Part model, mm, in its own coordinate system. Round coordinates to 2 decimals unless told otherwise and drop trailing zeros. Order: outer loops, then holes, each group sorted by start corner. A loop starts at its lowest first (then second) coordinate and runs counter-clockwise, first axis right, second up. Notation, with made-up numbers: (53, -8) -> (63, -8) arc R27 ccw to (63, 18) -> close; hole circle Ø2 at (59, -31.5). An arc over 180 degrees is marked (long way). Use CSV: the item, a comma, the result in double quotes.
```python
from build123d import *

# Parameters (mm, degrees)
F0_W     = 3.95
F0_H     = 6.85
F1_DEPTH = 2.425
F2_SIZE  = 0.8
F3_W     = 0.5
F3_H     = 0.5
F4_DEPTH = 6


with BuildPart() as f1:
    # F0 (on Front) → F1 (new body, symmetric)
    with BuildSketch(Plane.XZ):
        with Locations((0, 3.425)):
            Rectangle(F0_W, F0_H)
    extrude(amount=F1_DEPTH, both=True)

    # F2
    f2_edges = [f1.edges().sort_by_distance(p)[0] for p in [
        (0, 2.425, 6.85),
        (-1.975, -2.425, 3.425),
        (-1.975, 2.425, 3.425),
    ]]
    chamfer(f2_edges, length=F2_SIZE)

    # F3 (on face) → F4 (join)
    with BuildSketch(Plane(origin=(0, 0, 0), x_dir=(1, 0, 0), z_dir=(0, 0, -1))):
        with Locations((-0.275, 1.25)):
            Rectangle(F3_W, F3_H)
        with Locations((-0.275, -1.25)):
            Rectangle(F3_W, F3_H)
    extrude(amount=F4_DEPTH)


solid = f1.part
```
(1) Cut at C-C, the plane z = 1.5. Give the cut face in (x, y) (3 decimals).
Reply:
outline,"(-1.975, -1.625) -> (-1.175, -2.425) -> (1.975, -2.425) -> (1.975, 2.425) -> (-1.175, 2.425) -> (-1.975, 1.625) -> close"
(2) Cut at D-D, the plane y = -1.9. Give the cut face in (x, z) (3 decimals).
Reply:
outline,"(-1.7, 0) -> (1.975, 0) -> (1.975, 6.85) -> (-1.7, 6.85) -> close"
(3) Drop flat-ended pins along their axis: P1, Ø0.6, axis at x = -0.5, z = -1.5, coming from the +Y side; P2, Ø0.6, axis at x = 0, z = -2.5, coming from the -Y side; P3, Ø1.2, axis at x = 1, y = 0, coming from the -Z side. Give the stop position or say it passes through.
Reply:
P1,"y = 1.5"
P2,"y = -1.5"
P3,"z = 0"
(4) Cut at A-A, the plane z = -3.25. Give the cut face in (x, y) (3 decimals), then the cut area to 3 significant figures.
Reply:
outline,"(-0.525, -1.5) -> (-0.025, -1.5) -> (-0.025, -1) -> (-0.525, -1) -> close; (-0.525, 1) -> (-0.025, 1) -> (-0.025, 1.5) -> (-0.525, 1.5) -> close"
area,"0.500 mm2"
(5) Probe probe 1 along Y at (x, z) = (-0.45, -2); probe 2 along Z at (x, y) = (-1.7, 0.4); probe 3 along X at (y, z) = (-1.2, -2.5) (3 decimals). List the from-to ranges inside material, lowest first. Write a range as [from, to].
Reply:
probe 1,"[-1.5, -1], [1, 1.5]"
probe 2,"[0, 6.85]"
probe 3,"[-0.525, -0.025]"
(6) Cut at B-B, the plane x = 0.3. Give the cut face in (y, z) (3 decimals).
Reply:
outline,"(-2.425, 0) -> (2.425, 0) -> (2.425, 6.05) -> (1.625, 6.85) -> (-2.425, 6.85) -> close"
